from build123d import *

# Parameters (mm, degrees)
SKETCH1_R           = 2.85
BOSS_EXTRUDE1_DEPTH = 2
SKETCH2_R           = 1.5
BOSS_EXTRUDE2_DEPTH = 14
SKETCH3_W           = 6
SKETCH3_H           = 1
CUT_EXTRUDE1_DEPTH  = 1


with BuildPart() as part:
    # Sketch1 → Boss-Extrude1 (new body)
    with BuildSketch(Plane(origin=(0, 0, 0), x_dir=(1, 0, 0), z_dir=(0, 1, 0))):
        Circle(SKETCH1_R)
    extrude(amount=BOSS_EXTRUDE1_DEPTH)

    # Sketch2 → Boss-Extrude2 (add)
    with BuildSketch(Plane(origin=(0, 0, 0), x_dir=(1, 0, 0), z_dir=(0, 1, 0))):
        Circle(SKETCH2_R)
    extrude(amount=-BOSS_EXTRUDE2_DEPTH)

    # Sketch3 → Cut-Extrude1 (cut)
    with BuildSketch(Plane(origin=(0, 2, 0), x_dir=(1, 0, 0), z_dir=(0, 1, 0))):
        Rectangle(SKETCH3_W, SKETCH3_H)
    extrude(amount=-CUT_EXTRUDE1_DEPTH, mode=Mode.SUBTRACT)


solid = part.part
Geometry check sheet. Reference: the model listing, model coordinates, mm. A direction names the side the tool comes from. Round coordinates to 2 decimals unless told otherwise and drop trailing zeros. Loops run counter-clockwise (first coordinate to the right, second up) from the corner with the lowest first, then second, coordinate; pieces in that order, holes last. Notation, with made-up numbers: (62, 60.5) - (116, 60.5) arc R28 cw to (116, 94.5) - close; hole circle Ø2 at (4, 9.25). An arc over 180 degrees is marked (long way). One line per question, with ' | ' between items. Start each with the question number.
1. Tool access check on faces 1 (the face through (-1.5, -6.9, -0.07)), 2 (the face through (0, 1.5, -0.5)), 3 (the face through (0, 2, -1)). Record the directions out of +Z, -Z, +X, -X, +Y, -Y that give a thin tool (end or side, any length) a straight path to the whole face; none if there is none.
2. Cross-section at D-D on x = -1.8. Record the cut outline in (y, z), then the cut area to 3 significant figures.
3. Cross-section at B-B on z = 0. Record the cut outline in (x, y).
4. Scan lines: line 1 (Y direction, x = 1.9, z = 0.65); line 2 (X direction, y = -8, z = 0.05); line 3 (Y direction, x = -1.5, z = -0.3). Record each from-to range of solid material in increasing order. Write a range as [from, to].
5. Cross-section at A-A on x = 0. Record the cut outline in (y, z), then the cut area to 3 significant figures.
6. Depth check by flat-ended pin: pin 1 (2 mm diameter, centred on y = -8.5, z = -2, fed in from -X); pin 2 (0.5 mm diameter, centred on x = 0.5, z = 0, fed in from +Y); pin 3 (1 mm diameter, centred on x = -1.5, y = -1.5, fed in from -Z). Enter the tip coordinate at first touch or a pass-through.
7. Draft check along Z on faces 4 (the face through (0, -14, 0)), 5 (the face through (0, 1.5, 0.5)), 6 (the face through (2.633, 0.986, 1.092)). Enter one of: released by +Z, released by -Z, zero draft, split by the parting line, or undercut.
8. Cross-section at C-C on y = -5. Record the cut outline in (x, z).
Taken from the geometry:
1) face 1: -Y | face 2: +X, -X, +Y | face 3: +Z, -Z, +X, -X, +Y
2) outline: (0, -2.21) - (2, -2.21) - (2, -0.5) - (1, -0.5) - (1, 0.5) - (2, 0.5) - (2, 2.21) - (0, 2.21) - close | area: 7.84 mm²
3) outline: (-2.85, 0) - (-1.5, 0) - (-1.5, -14) - (1.5, -14) - (1.5, 0) - (2.85, 0) - (2.85, 1) - (-2.85, 1) - close
4) line 1: [0, 2] | line 2: [-1.5, 1.5] | line 3: [0, 1]
5) outline: (-14, -1.5) - (0, -1.5) - (0, -2.85) - (2, -2.85) - (2, -0.5) - (1, -0.5) - (1, 0.5) - (2, 0.5) - (2, 2.85) - (0, 2.85) - (0, 1.5) - (-14, 1.5) - close | area: 52.4 mm²
6) pin 1: x = -1.12 | pin 2: y = 1 | pin 3: z = -1.12
7) face 4: zero draft | face 5: undercut | face 6: split by the parting line
8) outline: circle Ø3 at (0, 0)
